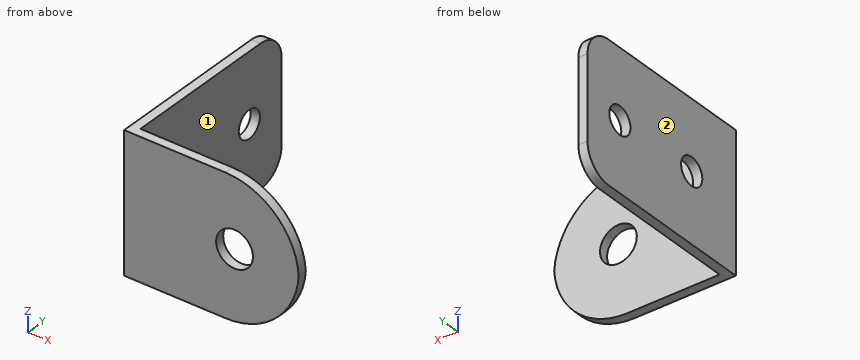
from build123d import *

# Parameters (mm, degrees)
EXTRUDE_THIN1_DEPTH = 15
FILLET1_R           = 8
SKETCH2_R           = 1.5
CUT_EXTRUDE1_DEPTH  = 32.391175729
FILLET2_R           = 3
SKETCH3_R           = 2
CUT_EXTRUDE2_DEPTH  = 31.796707523


with BuildPart() as part:
    # Sketch1 → Extrude-Thin1 (new body)
    with BuildSketch(Plane.XY):
        Polygon((18, 0), (0, 0), (0, 20), (-1, 20), (-1, -1), (18, -1), align=None)
    extrude(amount=EXTRUDE_THIN1_DEPTH)

    # Fillet1
    # the kernel refuses this fillet: 8 mm, written as the material it takes off along each edge
    with BuildSketch(Plane(origin=(18, -21, 0), x_dir=(0, 0, 1), z_dir=(0, 1, 0))) as fillet1_piece_1:
        with BuildLine():
            CenterArc((FILLET1_R, -FILLET1_R), FILLET1_R, 90, 90)
            Line((0, -FILLET1_R), (0, 0))
            Line((0, 0), (FILLET1_R, 0))
        make_face()
    extrude(amount=41, mode=Mode.SUBTRACT)
    with BuildSketch(Plane(origin=(18, -21, 15), x_dir=(0, 0, -1), z_dir=(0, 1, 0))) as fillet1_piece_2:
        with BuildLine():
            CenterArc((FILLET1_R, FILLET1_R), FILLET1_R, 180, 90)
            Line((0, FILLET1_R), (0, 0))
            Line((0, 0), (FILLET1_R, 0))
        make_face()
    extrude(amount=41, mode=Mode.SUBTRACT)

    # Sketch2 → Cut-Extrude1 (cut, through all)
    with BuildSketch(Plane.ZY.offset(1)):
        with Locations((7.5, 5.247627846)):
            Circle(SKETCH2_R)
        with Locations((7.5, 15.420132795)):
            Circle(SKETCH2_R)
    extrude(amount=-CUT_EXTRUDE1_DEPTH, mode=Mode.SUBTRACT)

    # Fillet2
    fillet2_edges = [part.edges().sort_by_distance(p)[0] for p in [
        (-0.5, 20, 15),
        (-0.5, 20, 0),
    ]]
    fillet(fillet2_edges, radius=FILLET2_R)

    # Sketch3 → Cut-Extrude2 (cut, through all)
    with BuildSketch(Plane(origin=(0, 0, 0), x_dir=(1, 0, 0), z_dir=(0, 1, 0))):
        with Locations(Location((11, -7.5, 0), (0, 0, 270))):
            Circle(SKETCH3_R)
    extrude(amount=-CUT_EXTRUDE2_DEPTH, mode=Mode.SUBTRACT)


solid = part.part
CAD build for the part. Positions are in the model's coordinates, mm. Face numbers are marked on the shaded views. A direction names the side the tool comes from. Round coordinates to 2 decimals unless told otherwise and drop trailing zeros. Write each loop counter-clockwise with the first axis right and the second up, starting at its lowest first coordinate (ties: lowest second). Pieces come first, ordered by that corner, then holes. Notation, with made-up numbers: M 69.5,-20 L 88.5,-20 A36 ccw 88.5,16 Z; hole C 74,-11 d2. An arc over 180 degrees is marked long. Use a Markdown table: item, result. Add a question column.
1. Drill centre lines: probe 1 along Y at (x, z) = (-0.7, 7.5); probe 2 along X at (y, z) = (9, 12). Where is each one in solid material? Low to high.
2. Flat gauge pins, fed straight in: P1, Ø5, axis at y = 5.25, z = 7.5, coming from the +X side; P2, Ø1.5, axis at x = 16, y = 1, coming from the +Z side. Where does each tip first touch, or does it go through?
3. Slice it at D-D on z = 1.5. Give the cut face in (x, y).
4. Slice it at A-A on y = 16.25. Give the cut face in (x, z).
5. 3-axis set-ups, long thin cutter, end or side, ignore diameter. For the marked faces 1 and 2: which of +Z, -Z, +X, -X, +Y, -Y reach the whole face in a straight line?
6. Slice it at B-B on x = 11. Give the cut face in (y, z).
7. Slice it at C-C on y = 9.25. Give the cut face in (x, z).
Reply:
| question | item | result |
|---|---|---|
| 1 | probe 1 | y = -1 to 3.75, 6.75 to 13.92, 16.92 to 20 |
| 1 | probe 2 | x = -1 to 0 |
| 2 | P1 | stops at x = 0 |
| 2 | P2 | passes through |
| 3 | outline | M -1,-1 L 14.66,-1 L 14.66,0 L 0,0 L 0,19.6 L -1,19.6 Z |
| 4 | outline | M -1,0 L 0,0 L 0,6.25 L -1,6.25 Z; M -1,8.75 L 0,8.75 L 0,15 L -1,15 Z |
| 5 | face 1 | +Z, -Z, +X, +Y |
| 5 | face 2 | +Z, -Z, -X, +Y, -Y |
| 6 | outline | M -1,0.06 L 0,0.06 L 0,5.5 L -1,5.5 Z; M -1,9.5 L 0,9.5 L 0,14.94 L -1,14.94 Z |
| 7 | outline | M -1,0 L 0,0 L 0,15 L -1,15 Z |
